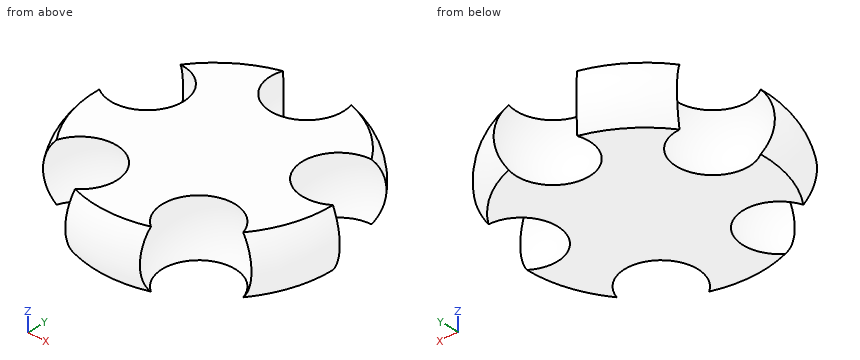
```python
from build123d import *

# Parameters (mm, degrees)
ARRAY_COUNT = 5


with BuildPart() as spheres:
    # Sphere → Sphere (revolve)
    with BuildSketch(Plane.XZ.offset(-22)):
        with BuildLine():
            ThreePointArc((0, -10), (10, 0), (0, 10))
            Line((0, 10), (0, -10))
        make_face()
    revolve(axis=Axis((0, 22, 0), (0, 0, 1)))

    # Array: spheres ×5 about axis
    array_axis = Axis((0, 0, 0), (0, 0, 1))


with BuildPart() as spheres_1:
    add(spheres.part)
    for i in range(1, ARRAY_COUNT):
        add(spheres.part.rotate(array_axis, i * 360 / ARRAY_COUNT))


with BuildPart() as hub_parametric:
    # Sketch → Revolution (revolve)
    with BuildSketch(Plane.YZ):
        with BuildLine():
            Line((-25.5, 6.2), (0, 6.2))
            Line((0, -6.2), (0, 6.2))
            Line((0, -6.2), (-25.5, -6.2))
            ThreePointArc((-25.5, 6.2), (-27.802084, 0), (-25.5, -6.2))
        make_face()
    revolve(axis=Axis((0, 0, 0), (0, 0, 1)))

    # Cut: cut spheres
    add(spheres_1.part, mode=Mode.SUBTRACT)


solid = hub_parametric.part
```
Check sheet for the modelled part. Datum: model origin and axes. Units: mm. Give positions to 0.01 mm unless a question says otherwise; leave off trailing zeros. Write each loop counter-clockwise with the first axis right and the second up, starting at its lowest first coordinate (ties: lowest second). Pieces come first, ordered by that corner, then holes.
Item 1: Cross-section at A-A (z = 4.5). Enter the section's corners in (x, y), and give its area (3 significant figures).
Item 2: Gauge pin test, flat ends, axial feed: pin 1 (2 mm diameter, centred on x = 21, z = -4, fed in from -Y); pin 2 (5 mm diameter, centred on x = -20.5, z = 1, fed in from +Y); pin 3 (2 mm diameter, centred on x = -10, z = 0.5, fed in from -Y). Record the tip position at first contact, or that the pin passes through.
Item 3: Cross-section at D-D (z = -0.5). Enter the section's corners in (x, y).
Item 4: Scan lines: L1, parallel to Y at x = 6.5, z = 5; L2, parallel to Y at x = -19, z = -1; L3, parallel to X at y = -12, z = 4.25. Record each from-to range of solid material in increasing order.
Item 5: Cross-section at C-C (y = 5.5). Enter the section's corners in (x, z), and give its area (3 significant figures).
Item 6: Cross-section at B-B (y = -12.5). Count the separate pieces of the cut face and the enclosed holes in it, and give its area (3 significant figures).
Report:
1. outline: (-26.67, -0.04) arc R26.67 ccw to (-21.6, -15.64) arc R8.93 cw (long way) to (-8.2, -25.38) arc R26.67 ccw to (8.2, -25.38) arc R8.93 cw (long way) to (21.6, -15.64) arc R26.67 ccw to (26.67, -0.04) arc R8.93 cw (long way) to (21.55, 15.71) arc R26.67 ccw to (8.28, 25.35) arc R8.93 cw (long way) to (-8.28, 25.35) arc R26.67 ccw to (-21.55, 15.71) arc R8.93 cw (long way) to start
1. area: 1,240 mm2
2. pin 1: stops at y = -15.74
2. pin 2: stops at y = 21.14
2. pin 3: stops at y = -8.62
3. outline: (-27.79, -0.46) arc R27.79 ccw to (-22.75, -15.96) arc R9.99 cw (long way) to (-8.15, -26.57) arc R27.79 ccw to (8.15, -26.57) arc R9.99 cw (long way) to (22.75, -15.96) arc R27.79 ccw to (27.79, -0.46) arc R9.99 cw (long way) to (22.21, 16.7) arc R27.79 ccw to (9.02, 26.28) arc R9.99 cw (long way) to (-9.02, 26.28) arc R27.79 ccw to (-22.21, 16.7) arc R9.99 cw (long way) to start
4. L1: y = -25.57 to -23.6, -12 to 16.28
4. L2: y = -9.91 to -2.96, 16.56 to 20.22
4. L3: x = -23.96 to -19.88, -5.98 to 5.98, 19.88 to 23.96
5. outline: (-13.19, -6.2) - (13.19, -6.2) arc R9.92 cw to (13.19, 6.2) - (-13.19, 6.2) arc R9.92 cw to start
5. area: 290 mm2
6. separate pieces: 3
6. enclosed holes: 0
6. area: 216 mm2
